Could you check a few things on this model? Use its own coordinates, in mm. Round coordinates to 2 decimals unless told otherwise and drop trailing zeros. Write each loop counter-clockwise with the first axis right and the second up, starting at its lowest first coordinate (ties: lowest second). Pieces come first, ordered by that corner, then holes. Notation, with made-up numbers: (14, -31) -> (59, -31) arc R12 ccw to (59, -26) -> close; hole circle Ø4 at (-31, 37). An arc over 180 degrees is marked (long way). One line per question, with ' | ' between items. Start each with the question number.
1. If I drill on line 1 along X through (y, z) = (-0.5, -12.75); line 2 along Z through (x, y) = (-35, 0.35); line 3 along Z through (x, y) = (35.5, -0.8), over which ranges is the centre line in solid material (lowest first)? Write a range as [from, to].
2. Imagine slicing it at B-B, the plane z = 0. List the corners of the cut face in (x, y) for me.
3. Imagine slicing it at C-C, the plane y = 0. State how many separate pieces and enclosed holes the cut face has, and give its area (3 significant figures).
4. Imagine slicing it at D-D, the plane z = 30. List the corners of the cut face in (x, y) for me.
5. For pin 1 Ø1.2 at (y, z) = (0.5, -32) entering from +X; pin 2 Ø4 at (x, z) = (35, 12.75) entering from +Y; pin 3 Ø2.5 at (x, z) = (15.25, -15.25) entering from -Y; pin 4 Ø0.8 at (y, z) = (-0.5, 33.5) entering from -X, each with a flat end and sliding along its axis, tell me the tip position at first contact or that it passes through.
6. Imagine slicing it at A-A, the plane x = -35. List the corners of the cut face in (y, z) for me.
from build123d import *

# Parameters (mm, degrees)
SKETCH1_W                  = 60
SKETCH1_H                  = 90
BOSS_EXTRUDE1_DEPTH        = 1.25
FILLET1_R                  = 3
F_4_2_4_2_DIAMETER_HOLE1_D = 4.2
M3_CLEARANCE_HOLE1_D       = 3.4


with BuildPart() as part:
    # Sketch1 → Boss-Extrude1 (new, symmetric)
    with BuildSketch(Plane(origin=(0, 0, 0), x_dir=(1, 0, 0), z_dir=(0, 1, 0))):
        Polygon((30, 45), (-30, 45), (-30, 25), (-30, -25), (-30, -45), (30, -45), (30, -25), (30, 25), align=None)
        Rectangle(SKETCH1_W, SKETCH1_H)
        Polygon((-30, -25), (-30, 25), (-39, 16), (-39, -16), align=None)
        Polygon((39, 16), (30, 25), (30, -25), (39, -16), align=None)
    extrude(amount=BOSS_EXTRUDE1_DEPTH, both=True)

    # Fillet1
    fillet1_edges = [part.edges().sort_by_distance(p)[0] for p in [
        (30, 0, -25),
        (39, 0, -16),
        (39, 0, 16),
        (30, 0, 25),
        (30, 0, 45),
        (-30, 0, 45),
        (-30, 0, 25),
        (-39, 0, 16),
        (-39, 0, -16),
        (-30, 0, -25),
        (-30, 0, -45),
        (30, 0, -45),
    ]]
    fillet(fillet1_edges, radius=FILLET1_R)

    # Ø4.2 (4.2) Diameter Hole1 (through all)
    with Locations(Plane(origin=(0, 1.25, 0), x_dir=(1, 0, 0), z_dir=(0, 1, 0))):
        with Locations((0, 0), (15.25, -15.25), (-15.25, 15.25), (-15.25, -15.25), (15.25, 15.25)):
            Hole(F_4_2_4_2_DIAMETER_HOLE1_D / 2)

    # M3 Clearance Hole1 (through all)
    with Locations(Plane(origin=(0, 1.25, 0), x_dir=(1, 0, 0), z_dir=(0, 1, 0))):
        with Locations((35, 12.75), (35, -12.75), (-35, -12.75), (-35, 12.75)):
            Hole(M3_CLEARANCE_HOLE1_D / 2)


solid = part.part
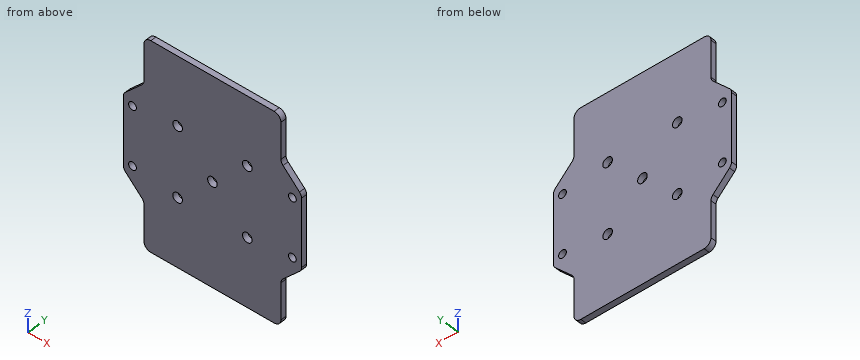
Geometry results:
1) line 1: x = [-39, -36.7], [-33.3, 33.3], [36.7, 39] | line 2: z = [-20, -14.45], [-11.05, 11.05], [14.45, 20] | line 3: z = [-19.5, -14.37], [-11.13, 11.13], [14.37, 19.5]
2) outline: (-39, -1.25) -> (-2.1, -1.25) -> (-2.1, 1.25) -> (-39, 1.25) -> close; (2.1, -1.25) -> (39, -1.25) -> (39, 1.25) -> (2.1, 1.25) -> close
3) separate pieces: 1 | enclosed holes: 9 | area: 6,020 mm2
4) outline: (-30, -1.25) -> (30, -1.25) -> (30, 1.25) -> (-30, 1.25) -> close
5) pin 1: stops at x = 30 | pin 2: stops at y = 1.25 | pin 3: passes through | pin 4: stops at x = -30
6) outline: (-1.25, -20) -> (1.25, -20) -> (1.25, -14.45) -> (-1.25, -14.45) -> close; (-1.25, -11.05) -> (1.25, -11.05) -> (1.25, 11.05) -> (-1.25, 11.05) -> close; (-1.25, 14.45) -> (1.25, 14.45) -> (1.25, 20) -> (-1.25, 20) -> close
